Study the drawing (mm; zero at the part's minimum x, y, z) and answer. A direction names the side the tool comes from. Round coordinates to 2 decimals unless told otherwise and drop trailing zeros. Write each loop counter-clockwise with the first axis right and the second up, starting at its lowest first coordinate (ties: lowest second). Pieces come first, ordered by that corner, then holes. Notation, with made-up numbers: (-16.5, 39.25) - (16.5, 39.25) arc R26 ccw to (16.5, 70.25) - close; hole circle Ø1 at (57, 54). An arc over 180 degrees is marked (long way). Return JSON: item names as keys, results as strings. Group by question number.
(1) Which of the six approach directions +Z, -Z, +X, -X, +Y, -Y give full straight-line access (tool end or side, diameter ignored) to the marked faces 1, 2, 3, 4 and 5?
(2) Section A-A, the plane y = 6 is taken. Write down the section's boundary in (x, z), then the cut area to 3 significant figures.
(3) Find the intervals of material crossed by line 1 along X through (y, z) = (6.5, 12); line 2 along X through (y, z) = (6.6, 33.5); line 3 along Y through (x, z) = (20, 18), in increasing order. Write a range as [from, to].
(4) Determine the mould class of the marked faces 6, 7, 8 and 9 for opening direction X: +X half, -X half, draft (parallel to the pull), parting line (faces both ways), or undercut.
(5) Section D-D, the plane y = 2 is taken. Write down the section's boundary in (x, z).
(6) Section C-C, the plane z = 12 is taken. Write down the section's boundary in (x, y), then the cut area to 3 significant figures.
(7) Each of these flat-tipped pins is pushed along its axis until it touches: pin 1 (2.5 mm diameter, centred on y = 6, z = 31, fed in from +X); pin 2 (1 mm diameter, centred on y = 2.5, z = 14.5, fed in from +X); pin 3 (4.5 mm diameter, centred on x = 32.4, z = 12, fed in from +Y). Where does it stop, or does it pass through?
(8) Section B-B, the plane x = 14.2 is taken. Write down the section's boundary in (y, z), then the cut area to 3 significant figures.
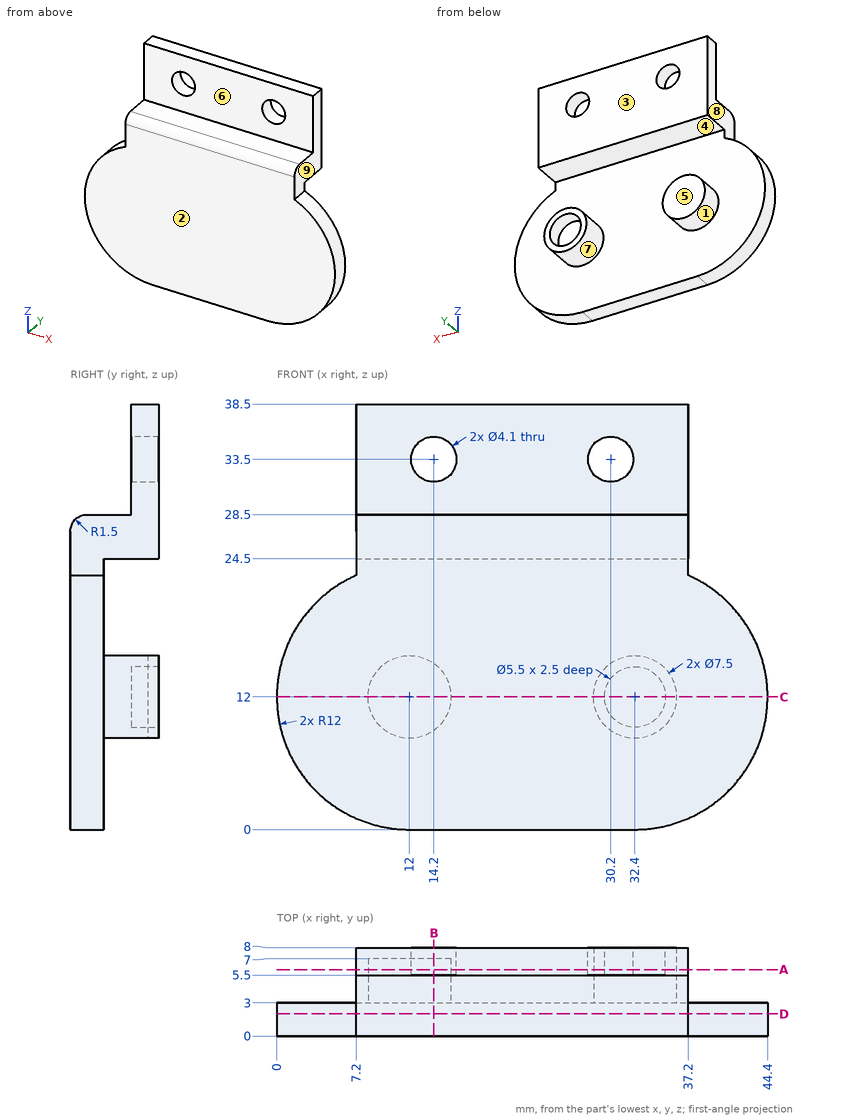
Working result:
{
 "1": {"face 1": "+Y", "face 2": "+Z, -Z, +X, -X, -Y", "face 3": "+Z, -Z, +X, -X, +Y", "face 4": "+X, -X, +Y", "face 5": "-Z, -X, +Y"},
 "2": {"outline": "(7.2, 24.5) - (37.2, 24.5) - (37.2, 38.5) - (7.2, 38.5) - close; circle Ø7.5 at (12, 12); circle Ø7.5 at (32.4, 12); hole circle Ø4.1 at (14.2, 33.5); hole circle Ø4.1 at (30.2, 33.5); hole circle Ø5.5 at (32.4, 12)", "area": "458 mm^2"},
 "3": {"line 1": "x = [8.25, 15.75], [28.65, 29.65], [35.15, 36.15]", "line 2": "x = [7.2, 12.15], [16.25, 28.15], [32.25, 37.2]", "line 3": "y = [0, 3]"},
 "4": {"face 6": "draft", "face 7": "undercut", "face 8": "-X half", "face 9": "+X half"},
 "5": {"outline": "(7.2, 23) arc R12 ccw to (12, 0) - (32.4, 0) arc R12 ccw to (37.2, 23) - (37.2, 28.5) - (7.2, 28.5) - close"},
 "6": {"outline": "(0, 0) - (44.4, 0) - (44.4, 3) - (36.15, 3) - (36.15, 8) - (35.15, 8) - (35.15, 5.5) - (29.65, 5.5) - (29.65, 8) - (28.65, 8) - (28.65, 3) - (15.75, 3) - (15.75, 7) - (8.25, 7) - (8.25, 3) - (0, 3) - close", "area": "187 mm^2"},
 "7": {"pin 1": "stops at x = 37.2", "pin 2": "stops at x = 44.23", "pin 3": "stops at y = 5.5"},
 "8": {"outline": "(0, 0) - (3, 0) - (3, 8.96) - (7, 8.96) - (7, 15.04) - (3, 15.04) - (3, 24.5) - (8, 24.5) - (8, 31.45) - (5.5, 31.45) - (5.5, 28.5) - (1.5, 28.5) arc R1.5 ccw to (0, 27) - close; (5.5, 35.55) - (8, 35.55) - (8, 38.5) - (5.5, 38.5) - close", "area": "144 mm^2"}
}
